Can you work these out from the model? Positions are in its coordinate system, mm. Round coordinates to 2 decimals unless told otherwise and drop trailing zeros. Order: outer loops, then holes, each group sorted by start corner. A loop starts at its lowest first (then second) coordinate and runs counter-clockwise, first axis right, second up.
Q1. Will these pins go through, and if not, where does the flat tip stop? P1, Ø5.5, axis at x = 193.35, y = 63.5, coming from the -Z side; P2, Ø0.5, axis at x = 17.5, z = 1, coming from the +Y side.
Q2. If we section it at A-A (x = 20): Please give me the cut outline in (y, z), plus the area to 3 significant figures.
Q3. If we section it at B-B (y = 215.9): Please give me the cut outline in (x, z).
Q4. If we section it at D-D (x = 193.35): Please give me the cut outline in (y, z), plus the area to 3 significant figures.
Q5. If we section it at C-C (z = 1.1): Count the separate pieces of the cut face and the enclosed holes in it, plus the area to 3 significant figures.
Q6. If I drill on line 1 (Y direction, x = 133.35, z = 0.75); line 2 (X direction, y = 31.75, z = 1.1); line 3 (Y direction, x = 194, z = 1.3), over which ranges is the centre line in solid material (lowest first)?
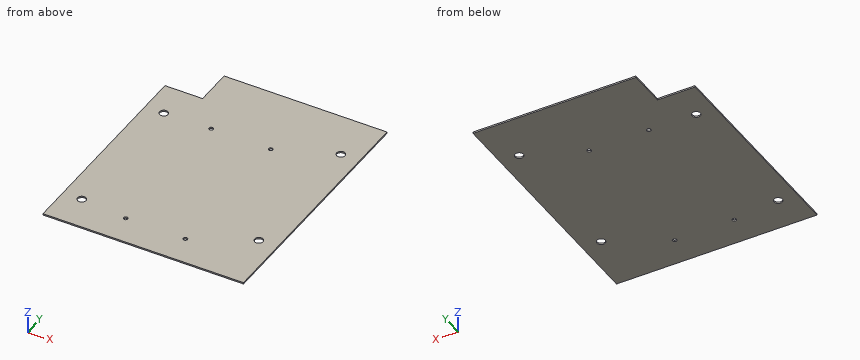
Autodesk Inventor part; units mm, degrees
ref_plane "YZ Plane" through (0, 0, 0) normal (1, 0, 0) x (0, 1, 0)
ref_plane "XZ Plane" through (0, 0, 0) normal (0, 1, 0) x (-1, 0, 0)
ref_plane "XY Plane" through (0, 0, 0) normal (0, 0, 1) x (1, 0, 0)
sketch "Sketch1" plane through (0, 0, 0) normal (0, 0, 1) x (1, 0, 0)
  line L0 (0, 0) -> (213.35, 0)
  line L1 (213.35, 0) -> (213.35, 266.7)
  line L2 (213.35, 266.7) -> (0, 266.7)
  line L3 (0, 266.7) -> (0, 0)
  line L4 (0, 0) -> (41.275, 0)
  line L5 (0, 41.275) -> (0, 0)
  line L6 (0, 266.7) -> (40, 266.7)
  line L7 (40, 266.7) -> (40, 226.7)
  line L8 (40, 226.7) -> (0, 226.7)
  line L9 (0, 226.7) -> (0, 266.7)
  dimension "d0" = 266.7
  dimension "d1" = 213.35
  dimension "d4" = 40
extrude "Extrusion1" add sketch "Sketch1" along normal blind 1.5875 contours L3 L8 L7 L2 L1 L0
sketch "Sketch2" plane through (0, 0, 1.5875) normal (0, 0, 1) x (1, 0, 0)
  line L0 (213.35, 0) -> (0, 0)
  line L1 (213.35, 266.7) -> (213.35, 0)
  line L2 (40, 266.7) -> (213.35, 266.7)
  line L3 (20, 189.55) -> (20, 37.15)
  line L4 (40, 266.7) -> (40, 226.7)
  line L5 (40, 266.7) -> (213.35, 266.7)
  line L6 (0, 0) -> (0, 226.7)
  line L7 (0, 226.7) -> (40, 226.7)
  line L8 (213.35, 266.7) -> (213.35, 0)
  line L9 (193.35, 215.9) -> (193.35, 63.5)
  point P0 (41.275, 0)
  point P1 (126.675, 266.7)
  point P2 (20, 113.35)
  point P3 (0, 113.35)
  dimension "d9" = 152.4
  dimension "d19" = 20
  dimension "d31" = 152.4
  dimension "d32" = 20
  dimension "d33" = 50.8
hole "Mounting Holes" at (20, 189.55, 1.5875) at (20, 37.15, 1.5875) at (193.35, 215.9, 1.5875) at (193.35, 63.5, 1.5875) direction (0, 0, -1) diameter 8.9916 end through all
sketch "Sketch3" plane through (0, 0, 1.5875) normal (0, 0, 1) x (1, 0, 0)
  line L0 (0, 0) -> (0, 226.7)
  line L1 (40, 266.7) -> (213.35, 266.7)
  line L2 (69.85, 190.5) -> (133.35, 190.5)
  line L3 (133.35, 190.5) -> (133.35, 31.75)
  line L4 (133.35, 31.75) -> (69.85, 31.75)
  line L5 (69.85, 31.75) -> (69.85, 190.5)
  dimension "d20" = 69.85
  dimension "d21" = 63.5
  dimension "d22" = 158.75
  dimension "d23" = 76.2
hole "PSU Mounting Holes" at (69.85, 190.5, 1.5875) at (133.35, 190.5, 1.5875) at (69.85, 31.75, 1.5875) at (133.35, 31.75, 1.5875) direction (0, 0, -1) diameter 4.4958 end through all
properties part number "front right plate" material "Aluminum-6061"
Solution:
1. P1: passes through
1. P2: stops at y = 226.7
2. outline: (0, 0) - (32.65, 0) - (32.65, 1.59) - (0, 1.59) - close; (41.65, 0) - (185.05, 0) - (185.05, 1.59) - (41.65, 1.59) - close; (194.05, 0) - (226.7, 0) - (226.7, 1.59) - (194.05, 1.59) - close
2. area: 331 mm2
3. outline: (0, 0) - (188.85, 0) - (188.85, 1.59) - (0, 1.59) - close; (197.85, 0) - (213.35, 0) - (213.35, 1.59) - (197.85, 1.59) - close
4. outline: (0, 0) - (59, 0) - (59, 1.59) - (0, 1.59) - close; (68, 0) - (211.4, 0) - (211.4, 1.59) - (68, 1.59) - close; (220.4, 0) - (266.7, 0) - (266.7, 1.59) - (220.4, 1.59) - close
4. area: 395 mm2
5. separate pieces: 1
5. enclosed holes: 8
5. area: 55,000 mm2
6. line 1: y = 0 to 29.5, 34 to 188.25, 192.75 to 266.7
6. line 2: x = 0 to 67.6, 72.1 to 131.1, 135.6 to 213.35
6. line 3: y = 0 to 59.05, 67.95 to 211.45, 220.35 to 266.7
